Build history of the part. All positions in model axes, mm. Give positions to 0.01 mm unless a question says otherwise; leave off trailing zeros. Order: outer loops, then holes, each group sorted by start corner. A loop starts at its lowest first (then second) coordinate and runs counter-clockwise, first axis right, second up. Notation, with made-up numbers: (38, 45) - (97, 45) arc R13 ccw to (97, 67) - close; hole circle Ø10 at (40, 23). An arc over 180 degrees is marked (long way). Answer in a Markdown table with one row per item.
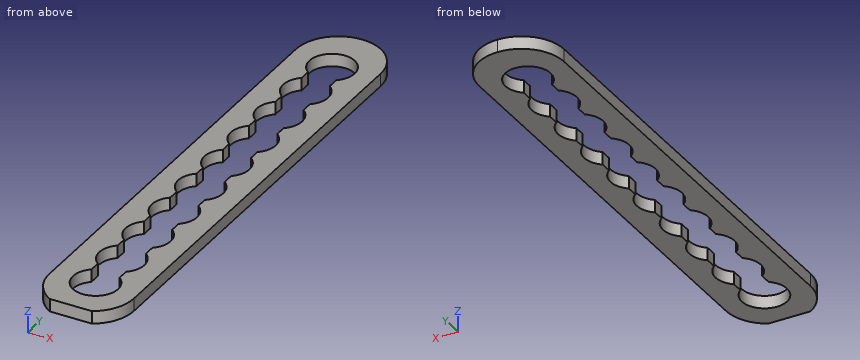
```python
from build123d import *

# Parameters (mm, degrees)
CROQUIS1_W              = 30
CROQUIS1_H              = 185
SALIENTE_EXTRUIR1_DEPTH = 4.5
REDONDEO1_R             = 15
CROQUIS2_R              = 8
CORTAR_EXTRUIR1_DEPTH   = 10
CROQUIS3_W              = 36.075387002
CROQUIS3_H              = 11.559576231
CORTAR_EXTRUIR2_DEPTH   = 10


with BuildPart() as part:
    # Croquis1 → Saliente-Extruir1 (new body)
    with BuildSketch(Plane.XY):
        Rectangle(CROQUIS1_W, CROQUIS1_H)
        with BuildLine():
            Line((5, 72.5), (5, -72.5))
            ThreePointArc((5, -72.5), (0, -77.5), (-5, -72.5))
            Line((-5, -72.5), (-5, 72.5))
            ThreePointArc((-5, 72.5), (0, 77.5), (5, 72.5))
        make_face(mode=Mode.SUBTRACT)
    extrude(amount=SALIENTE_EXTRUIR1_DEPTH)

    # Redondeo1
    redondeo1_edges = [part.edges().sort_by_distance(p)[0] for p in [
        (15, -92.5, 2.25),
        (-15, -92.5, 2.25),
        (-15, 92.5, 2.25),
        (15, 92.5, 2.25),
    ]]
    fillet(redondeo1_edges, radius=REDONDEO1_R - 0.0001)  # a hair under: the kernel refuses the full size

    # Croquis2 → Cortar-Extruir1 (cut)
    with BuildSketch(Plane.XY.offset(4.5)):
        with Locations((0, 73.5)):
            Circle(CROQUIS2_R)
        with Locations((0, 57)):
            Circle(CROQUIS2_R)
        with Locations((0, 40.5)):
            Circle(CROQUIS2_R)
        with Locations((0, 24)):
            Circle(CROQUIS2_R)
        with Locations((0, 7.5)):
            Circle(CROQUIS2_R)
        with Locations((0, -9)):
            Circle(CROQUIS2_R)
        with Locations((0, -25.5)):
            Circle(CROQUIS2_R)
        with Locations((0, -42)):
            Circle(CROQUIS2_R)
        with Locations((0, -58.5)):
            Circle(CROQUIS2_R)
        with Locations((0, -75)):
            Circle(CROQUIS2_R)
    extrude(amount=-CORTAR_EXTRUIR1_DEPTH, mode=Mode.SUBTRACT)

    # Croquis3 → Cortar-Extruir2 (cut)
    with BuildSketch(Plane.XY.offset(4.5)):
        with Locations((0.166198184, -96.279788115)):
            Rectangle(CROQUIS3_W, CROQUIS3_H)
    extrude(amount=-CORTAR_EXTRUIR2_DEPTH, mode=Mode.SUBTRACT)


solid = part.part
```
1. Drop flat-ended pins along their axis: P1, Ø2, axis at x = 8, z = 2.5, coming from the +Y side; P2, Ø1.5, axis at x = 10, z = 2.5, coming from the -Y side. Give the stop position or say it passes through.
Check result:
| item | result |
|---|---|
| P1 | stops at y = 90.77 |
| P2 | stops at y = -89.31 |
2. Cut at A-A on y = 73.5. Write the cut outline in (x, z).
Check result:
| item | result |
|---|---|
| outline | (-15, 0) - (-8, 0) - (-8, 4.5) - (-15, 4.5) - close; (8, 0) - (15, 0) - (15, 4.5) - (8, 4.5) - close |
3. Cut at C-C on x = 13.5. Write the cut outline in (y, z).
Check result:
| item | result |
|---|---|
| outline | (-84.04, 0) - (84.04, 0) - (84.04, 4.5) - (-84.04, 4.5) - close |
4. Probe line 1 (Y direction, x = 0, z = 3); line 2 (X direction, y = -75, z = 2.3); line 3 (X direction, y = -32.5, z = 1.4). List the from-to ranges inside material, lowest first.
Check result:
| item | result |
|---|---|
| line 1 | y = -90.5 to -83, 81.5 to 92.5 |
| line 2 | x = -15 to -8, 8 to 15 |
| line 3 | x = -15 to -5, 5 to 15 |
5. Cut at B-B on x = -3. Write the cut outline in (y, z).
Check result:
| item | result |
|---|---|
| outline | (-90.5, 0) - (-82.42, 0) - (-82.42, 4.5) - (-90.5, 4.5) - close; (80.92, 0) - (92.2, 0) - (92.2, 4.5) - (80.92, 4.5) - close |
